Source: CAD feature listing. Evaluate the final solid. Frame: model axes, mm. A direction names the side the tool comes from. Give positions to 0.01 mm unless a question says otherwise; leave off trailing zeros. Loops run counter-clockwise (first coordinate to the right, second up) from the corner with the lowest first, then second, coordinate; pieces in that order, holes last. Notation, with made-up numbers: M 4.25,17.25 L 37.25,17.25 A19 ccw 37.25,35.25 Z; hole C 41,86.5 d7. An arc over 180 degrees is marked long. Put each result on its own line as item: value.
from build123d import *

# Parameters (mm, degrees)
F0_R      = 19.05
F1_DEPTH  = 17.4625
F2_R      = 8.7141687226
F3_DEPTH  = 37.084
F4_R      = 12.7
F5_DEPTH  = 5.08
F6_R      = 5.3581350259
F7_DEPTH  = 31.75
F10_W     = 6.35
F10_H     = 5.08
F11_DEPTH = 3.175


with BuildPart() as f1:
    # F0 (on Front) → F1 (new body, symmetric)
    with BuildSketch(Plane.XZ):
        Circle(F0_R)
    extrude(amount=F1_DEPTH, both=True)

    # F2 (on face) → F3 (join)
    with BuildSketch(Plane.XZ.offset(17.4625)):
        Circle(F2_R)
    extrude(amount=F3_DEPTH)

    # F4 (on face) → F5 (join)
    with BuildSketch(Plane(origin=(0, 17.4625, 0), x_dir=(-1, 0, 0), z_dir=(0, 1, 0))):
        Circle(F4_R)
    extrude(amount=F5_DEPTH)

    # F6 (on face) → F7 (cut)
    with BuildSketch(Plane(origin=(0, 22.5425, 0), x_dir=(-1, 0, 0), z_dir=(0, 1, 0))):
        Circle(F6_R)
    extrude(amount=-F7_DEPTH, mode=Mode.SUBTRACT)

    # F10 (on plane+point) → F11 (cut)
    with BuildSketch(Plane.XY.offset(12.7)):
        with Locations((0, 20.0025)):
            Rectangle(F10_W, F10_H)
    extrude(amount=-F11_DEPTH, mode=Mode.SUBTRACT)


solid = f1.part
1. Access query for faces 4 (the flat face through (0, -9.208, 0)), 5 (the flat face through (3.175, 20, 11)), 6 (the flat face through (0, 22.542, -6)), 7 (the cylindrical face through (8.31, -35.74, 2.62)). Directions: +Z, -Z, +X, -X, +Y, -Y. A direction counts if a zero-diameter tool reaches every point of the face in a straight line with its end or side. Return the directions, or none.
Found:
face 4: +Y
face 5: +Z, +Y
face 6: +Z, -Z, +X, -X, +Y
face 7: -Y
2. Section query C-C (y = -1). Output: boundary loops of the cut face in (x, z).
Found:
outline: C 0,0 d38.1; hole C 0,0 d10.72
3. Material intervals for line 1 (Z direction, x = 0, y = 2); line 2 (Y direction, x = -0.5, z = 15.5); line 3 (Y direction, x = -4, z = -3.5), sorted ascending. Write a range as from..to.
Found:
line 1: -19.05..-5.36, 5.36..19.05
line 2: -17.46..17.46
line 3: -54.55..-9.21
4. Section query D-D (y = -38.5). Output: boundary loops of the cut face in (x, z).
Found:
outline: C 0,0 d17.43
5. Section query B-B (z = 0). Output: boundary loops of the cut face in (x, y), plus the area to 3 significant figures.
Found:
outline: M -19.05,-17.46 L -8.71,-17.46 L -8.71,-54.55 L 8.71,-54.55 L 8.71,-17.46 L 19.05,-17.46 L 19.05,17.46 L 12.7,17.46 L 12.7,22.54 L 5.36,22.54 L 5.36,-9.21 L -5.36,-9.21 L -5.36,22.54 L -12.7,22.54 L -12.7,17.46 L -19.05,17.46 Z
area: 1,770 mm^2
6. Contact query for flat-ended pins moving along their axis: P1, Ø12, axis at x = -7, y = -33, coming from the -Z side; P2, Ø10, axis at y = -28.5, z = -1, coming from the +X side; P3, Ø1.5, axis at x = -1, y = 21, coming from the +Z side (3 decimals). Output: stop coordinate, or through.
Found:
P1: z = -8.66
P2: x = 8.71
P3: z = 9.525
7. Draft query along X for faces 1 (the cylindrical face through (-15.12, -0.24, -11.59)), 2 (the flat face through (8, -17.462, -4)), 3 (the flat face through (0, 20, 9.525)). Return one class per face: pulls with the +X half, pulls with the -X half, needs draft (parallel to the pull), parting line crosses it, or undercut.
Found:
face 1: parting line crosses it
face 2: needs draft
face 3: undercut
